from build123d import *

# Parameters (mm, degrees)
FILLET1_R = 0.5


with BuildPart() as part:
    # Sketch1 → Revolve1 (revolve)
    with BuildSketch(Plane.XY):
        Polygon((-1.55, 0), (-7, 0), (-7, -5.5), (-4, -5.5), (-4, -3.373831776), (-1.55, -3.373831776), align=None)
    revolve(axis=Axis((0, 0, 0), (0, 1, 0)))

    # Fillet1
    fillet1_edges = [part.edges().sort_by_distance(p)[0] for p in [
        (4, -5.5, 0),
        (7, -5.5, 0),
    ]]
    fillet(fillet1_edges, radius=FILLET1_R)


solid = part.part
Here's how the part is built. I have some questions about the finished solid (model axes, mm). A direction names the side the tool comes from. Round coordinates to 2 decimals unless told otherwise and drop trailing zeros. Write each loop counter-clockwise with the first axis right and the second up, starting at its lowest first coordinate (ties: lowest second). Pieces come first, ordered by that corner, then holes.
1. Suppose I cut it at A-A (x = 0). List the corners of the cut face in (y, z) for me, and give its area (3 significant figures).
2. Will these pins go through, and if not, where does the flat tip stop? pin 1 Ø6 at (x, z) = (1.5, -2) entering from -Y; pin 2 Ø4 at (x, z) = (0.5, 1) entering from -Y; pin 3 Ø1 at (y, z) = (-2, 3.5) entering from -X; pin 4 Ø1.5 at (y, z) = (-4, -4.5) entering from -X.
3. Suppose I cut it at C-C (y = -2.5). List the corners of the cut face in (x, z) for me.
4. For faces 1 (the cylindrical face through (0.867, -4.176, -3.905)), 2 (the flat face through (1.54, -5.5, 4.42)), which set-ups out of +Z, -Z, +X, -X, +Y, -Y let a thin tool reach every point of the face, with its end or its side?
5. If we mould it in two halves opening along Z, with no side actions, what happens to faces 3 (the flat face through (-2, -3.374, 0)), 4 (the flat face through (0, 0, 2)), 5 (the cylindrical face through (-6.466, -2.535, -2.681))? For each: released by +Z, released by -Z, zero draft, split by the parting line, or undercut.
6. I need wall thicknesses on L1, parallel to Z at x = 0, y = -2.6; L2, parallel to Y at x = 2, z = 0.75; L3, parallel to Z at x = 0, y = -3.65. Which ranges of each line are inside material? Lowest first, please.
7. Suppose I cut it at B-B (z = 0). List the corners of the cut face in (x, y) for me.
Answer sheet:
1. outline: (-5.5, -6.5) arc R0.5 ccw to (-5, -7) - (0, -7) - (0, -1.55) - (-3.37, -1.55) - (-3.37, -4) - (-5, -4) arc R0.5 ccw to (-5.5, -4.5) - close; (-5.5, 4.5) arc R0.5 ccw to (-5, 4) - (-3.37, 4) - (-3.37, 1.55) - (0, 1.55) - (0, 7) - (-5, 7) arc R0.5 ccw to (-5.5, 6.5) - close
1. area: 49.3 mm2
2. pin 1: stops at y = -5.5
2. pin 2: stops at y = -3.37
2. pin 3: stops at x = -6.32
2. pin 4: stops at x = -5.91
3. outline: circle Ø14 at (0, 0); hole circle Ø3.1 at (0, 0)
4. face 1: -Y
4. face 2: +Z, -Z, +X, -X, -Y
5. face 3: undercut
5. face 4: zero draft
5. face 5: split by the parting line
6. L1: z = -7 to -1.55, 1.55 to 7
6. L2: y = -3.37 to 0
6. L3: z = -7 to -4, 4 to 7
7. outline: (-7, -5) arc R0.5 ccw to (-6.5, -5.5) - (-4.5, -5.5) arc R0.5 ccw to (-4, -5) - (-4, -3.37) - (-1.55, -3.37) - (-1.55, 0) - (-7, 0) - close; (1.55, -3.37) - (4, -3.37) - (4, -5) arc R0.5 ccw to (4.5, -5.5) - (6.5, -5.5) arc R0.5 ccw to (7, -5) - (7, 0) - (1.55, 0) - close
